from build123d import *

# Parameters (mm, degrees)
BOSS_EXTRU_1_DEPTH                = 48
DIAM_TRE_DU_PER_AGE_3_0_3_1_D     = 3
DIAM_TRE_DU_PER_AGE_3_0_3_1_DEPTH = 10
DIAM_TRE_DU_PER_AGE_2_0_2_1_D     = 2
DIAM_TRE_DU_PER_AGE_2_0_2_1_DEPTH = 9.000001526
DIAM_TRE_DU_PER_AGE_3_0_3_2_D     = 3
DIAM_TRE_DU_PER_AGE_3_0_3_2_DEPTH = 9.000001526


with BuildPart() as part:
    # Esquisse1 → Boss.-Extru.1 (new body)
    with BuildSketch(Plane(origin=(79.448008992, 0, -79.44794681), x_dir=(0, 1, 0), z_dir=(0.7071070579059934, 0, -0.7071065044669933))):
        with BuildLine():
            Line((188.763426925, 171.056630761), (157.836573075, 171.056630761))
            ThreePointArc((157.836573075, 171.056630761), (154.773801793, 168.43282973), (152.150000763, 165.370058448))
            Line((152.150000763, 165.370058448), (152.150000763, 134.443204599))
            ThreePointArc((152.150000763, 134.443204599), (154.77380225, 131.38043286), (157.836574119, 128.756631524))
            Line((157.836574119, 128.756631524), (188.763425881, 128.756631524))
            ThreePointArc((188.763425881, 128.756631524), (191.826198207, 131.380433317), (194.45, 134.443205643))
            Line((194.45, 134.443205643), (194.45, 165.370057405))
            ThreePointArc((194.45, 165.370057405), (191.826198664, 168.432829273), (188.763426925, 171.056630761))
        make_face()
    extrude(amount=-BOSS_EXTRU_1_DEPTH)

    # Esquisse2 → Révolution1 (revolve)
    with BuildSketch(Plane(origin=(0, 173.3, 0), x_dir=(1, 0, 0), z_dir=(0, 1, 0))):
        Polygon((164.213527842, -73.19991591), (151.506824443, -60.493202565), (103.989230421, -108.010759396), (106.817656439, -110.839187627), (119.828426035, -97.828428215), (124.778171566, -102.77817762), (126.12167388, -101.434676357), (131.050205731, -106.363212066), align=None)
    revolve(axis=Axis((132.687188584, 173.3, 79.312823694), (-0.7071070579059953, 0, 0.7071065044669914)))

    # Diamètre du perçage Ø3.0 (3)1
    with Locations(Plane(origin=(45.506870213, 0, -45.506834595), x_dir=(0.7071065044669932, 0, 0.7071070579059936), z_dir=(-0.7071070579059936, 0, 0.7071065044669932))):
        with Locations((134.406631524, 188.8), (134.406631524, 157.8), (165.406631524, 188.8), (165.406631524, 157.8)):
            Hole(DIAM_TRE_DU_PER_AGE_3_0_3_1_D / 2, depth=DIAM_TRE_DU_PER_AGE_3_0_3_1_DEPTH)

    # Diamètre du perçage Ø2.0 (2)1
    with Locations(Plane(origin=(12.343548118, 0, -12.343538457), x_dir=(0.7071065044669916, 0, 0.7071070579059952), z_dir=(-0.7071070579059952, 0, 0.7071065044669916))):
        with Locations((149.906631524, 159.2), (164.006631524, 173.3), (135.806631524, 173.3), (149.906631524, 187.4)):
            Hole(DIAM_TRE_DU_PER_AGE_2_0_2_1_D / 2, depth=DIAM_TRE_DU_PER_AGE_2_0_2_1_DEPTH)

    # Diamètre du perçage Ø3.0 (3)2
    with Locations(Plane(origin=(12.343548118, 0, -12.343538457), x_dir=(0.7071065044669916, 0, 0.7071070579059952), z_dir=(-0.7071070579059952, 0, 0.7071065044669916))):
        with Locations((139.906631524, 163.3), (139.906631524, 183.3), (159.906631524, 183.3), (159.906631524, 163.3)):
            Hole(DIAM_TRE_DU_PER_AGE_3_0_3_2_D / 2, depth=DIAM_TRE_DU_PER_AGE_3_0_3_2_DEPTH)


solid = part.part
Source: CAD feature listing. Evaluate the final solid. Frame: model axes, mm. A direction names the side the tool comes from. Coordinates: 2 decimals unless noted, no trailing zeros. Loops run counter-clockwise (first coordinate to the right, second up) from the corner with the lowest first, then second, coordinate; pieces in that order, holes last. Notation, with made-up numbers: (58, 37) -> (89, 37) arc R25 ccw to (89, 59) -> close; hole circle Ø6 at (83.5, 49.5). An arc over 180 degrees is marked (long way). Answer in a Markdown table with one row per item. Add a question column.
Q1. Section B-B on x = 112. Give the number of separate pieces and of enclosed holes in the cut face, and give its area (3 significant figures).
Q2. Contact query for flat-ended pins moving along their axis: pin 1 Ø5 at (x, y) = (113, 181) entering from -Z; pin 2 Ø5 at (x, y) = (187, 163) entering from -Z; pin 3 Ø2 at (x, y) = (131, 182.5) entering from -Z. Output: stop coordinate, or through.
Q3. Section C-C on y = 175.5. Return the cut outline in (x, z), and give its area (3 significant figures).
Q4. Pull-direction query (Y, two-part tool) for faces 3 (the face through (111.89, 169.75, 102.72)), 4 (the face through (111.69, 174.29, 80.55)), 5 (the face through (128.871, 161.836, 97.731)), 6 (the face through (104.03, 173.36, 108.05)); classes: pulls with the +Y half, pulls with the -Y half, needs draft (parallel to the pull), parting line crosses it, or undercut.
Q5. Reachability of faces 1 (the face through (124.169, 165.565, 99.482)), 2 (the face through (185.657, 173.004, 26.761)) from +Z, -Z, +X, -X, +Y, -Y: full face, straight path, thin tool, end or side. Return the list, or none.
Q6. Ray query, line 1 along Z through (x, y) = (140, 158.5); line 2 along Z through (x, y) = (109, 174.5); line 3 along Y through (x, z) = (138.5, 54). Return the intervals inside material, ascending.
Q7. Section A-A on y = 166. Return the cut outline in (x, z) (1 decimal).
Computed values:
| question | item | result |
|---|---|---|
| 1 | separate pieces | 2 |
| 1 | enclosed holes | 1 |
| 1 | area | 370 mm^2 |
| 2 | pin 1 | stops at z = 73.11 |
| 2 | pin 2 | stops at z = 25.6 |
| 2 | pin 3 | stops at z = 57.89 |
| 3 | outline | (101.63, 105.65) -> (114.64, 92.64) -> (109.38, 87.38) -> (110.72, 86.04) -> (105.73, 81.05) -> (138.9, 47.88) -> (136.55, 45.54) -> (170.49, 11.6) -> (200.4, 41.51) -> (166.46, 75.45) -> (164.12, 73.1) -> (130.95, 106.27) -> (125.96, 101.28) -> (124.62, 102.62) -> (119.36, 97.36) -> (106.35, 110.37) -> close |
| 3 | area | 3,870 mm^2 |
| 4 | face 3 | parting line crosses it |
| 4 | face 4 | undercut |
| 4 | face 5 | undercut |
| 4 | face 6 | needs draft |
| 5 | face 1 | none |
| 5 | face 2 | -Z, +X, +Y, -Y |
| 6 | line 1 | z = 42.09 to 48.2, 57.59 to 86.41 |
| 6 | line 2 | z = 77.64 to 84.31, 97.6 to 108.4 |
| 6 | line 3 | y = 161.78 to 184.82 |
| 7 | outline | (106.7, 82) -> (139.9, 48.9) -> (136.6, 45.5) -> (170.5, 11.6) -> (200.4, 41.5) -> (166.5, 75.4) -> (163.1, 72.1) -> (130, 105.3) -> (124.2, 99.5) -> (122.8, 100.8) -> (111.2, 89.2) -> (112.5, 87.8) -> close |
